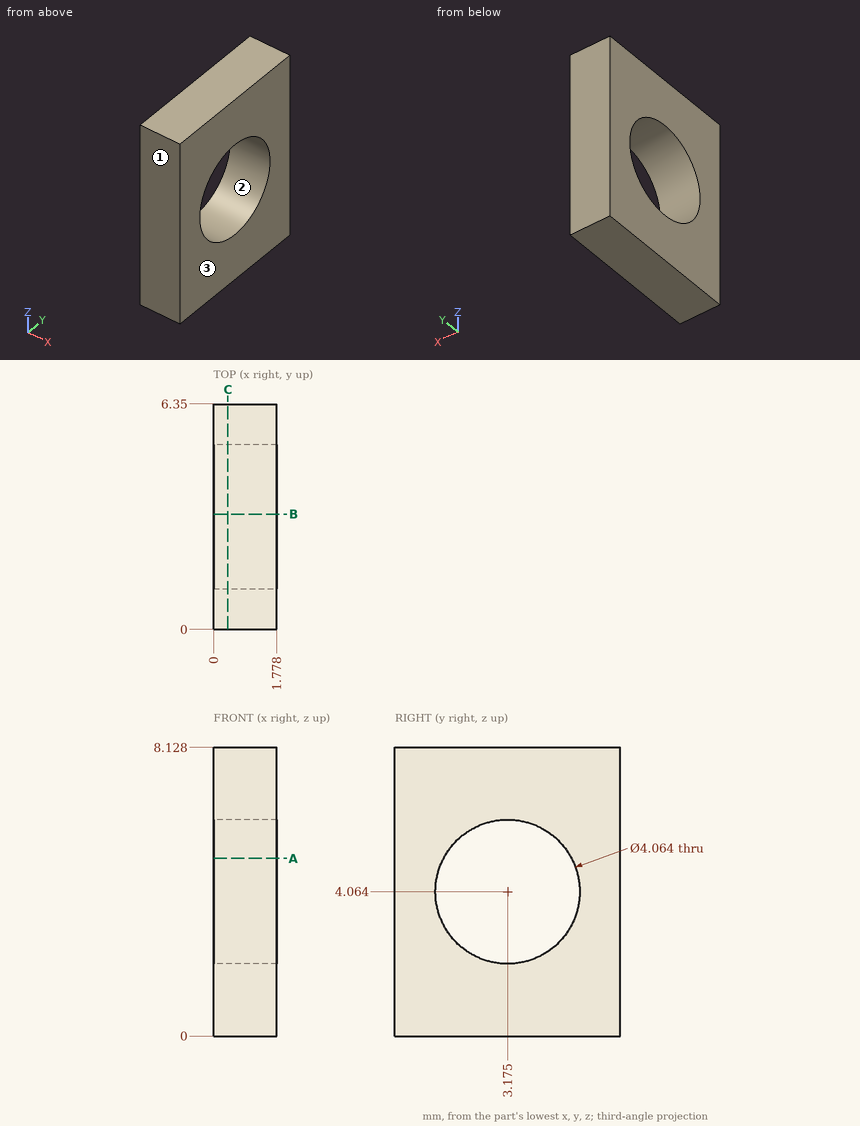
Job drawing, mm, ordinate dimensions from the low corner. One solid piece. Coordinates: 2 decimals unless noted, no trailing zeros. Order: outer loops, then holes, each group sorted by start corner. A loop starts at its lowest first (then second) coordinate and runs counter-clockwise, first axis right, second up. Notation, with made-up numbers: (-25.75, 42.5) -> (29.25, 42.5) arc R13 ccw to (29.25, 65.5) -> close; hole circle Ø3 at (66, 57). An arc over 180 degrees is marked (long way). Put each result on its own line as item: value. Start each with the question number.
(1) Probe line 1 along Z through (x, y) = (0.2, 3.25); line 2 along Y through (x, z) = (0.85, 4); line 3 along Y through (x, z) = (0.9, 3.5). List the from-to ranges inside material, lowest first. Write a range as [from, to].
(2) Band-saw the part on A-A (z = 5). Give the cut face in (x, y), then the cut area to 3 significant figures.
(3) Mould opens along Y. For the marked faces 1, 2 and 3 say: pulls with the +Y half, pulls with the -Y half, needs draft (parallel to the pull), parting line crosses it, or undercut.
(4) Band-saw the part on C-C (x = 0.4). Give the cut face in (y, z) (3 decimals).
(5) Band-saw the part on B-B (y = 3.25). Give the cut face in (x, z).
Determined:
1. line 1: z = [0, 2.03], [6.09, 8.13]
1. line 2: y = [0, 1.14], [5.21, 6.35]
1. line 3: y = [0, 1.22], [5.13, 6.35]
2. outline: (0, 0) -> (1.78, 0) -> (1.78, 1.37) -> (0, 1.37) -> close; (0, 4.98) -> (1.78, 4.98) -> (1.78, 6.35) -> (0, 6.35) -> close
2. area: 4.88 mm²
3. face 1: pulls with the -Y half
3. face 2: undercut
3. face 3: needs draft
4. outline: (0, 0) -> (6.35, 0) -> (6.35, 8.128) -> (0, 8.128) -> close; hole circle Ø4.064 at (3.175, 4.064)
5. outline: (0, 0) -> (1.78, 0) -> (1.78, 2.03) -> (0, 2.03) -> close; (0, 6.09) -> (1.78, 6.09) -> (1.78, 8.13) -> (0, 8.13) -> close
